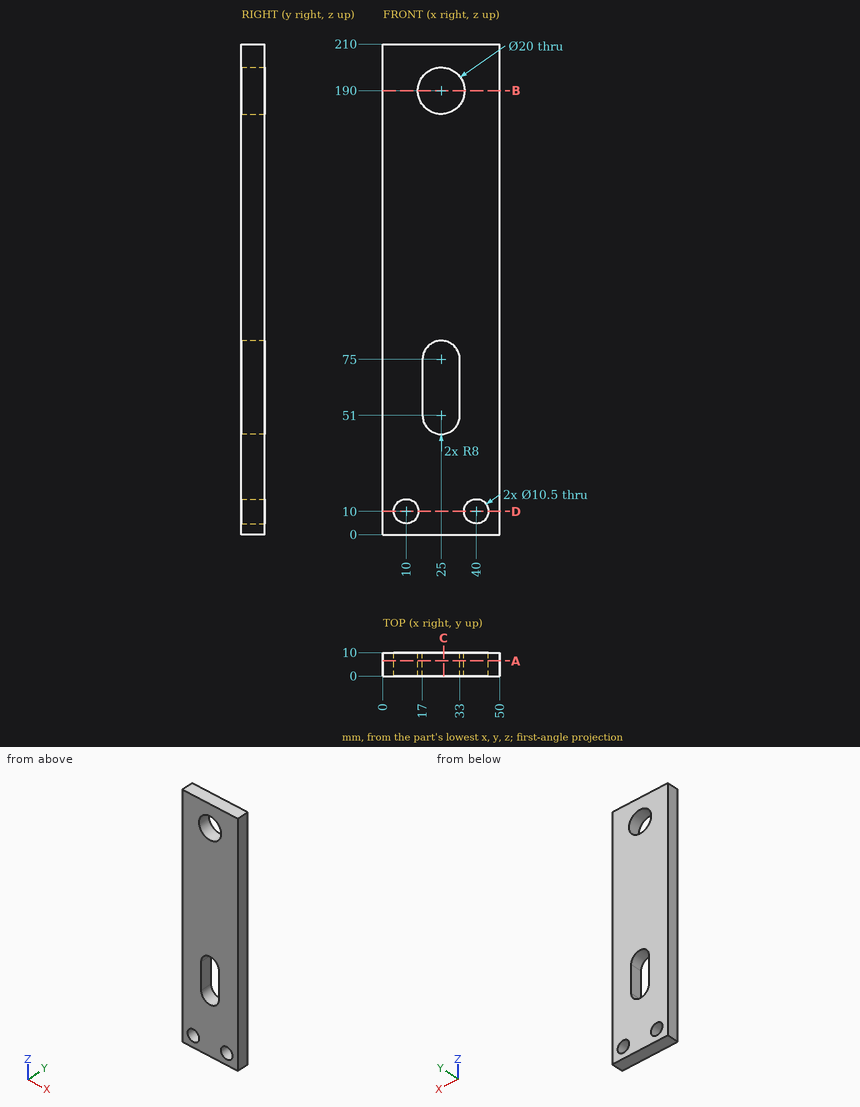
Answer from the drawing. Dimensions are ordinates in mm from the lowest x, y and z of the part. Give positions to 0.01 mm unless a question says otherwise; leave off trailing zeros. Loops run counter-clockwise (first coordinate to the right, second up) from the corner with the lowest first, then second, coordinate; pieces in that order, holes last. Notation, with made-up numbers: (-2, 84.5) -> (6, 84.5) arc R18 ccw to (6, 97.5) -> close; hole circle Ø2 at (35.25, 80.5). An arc over 180 degrees is marked (long way). One line per question, with ' | ' between items. Start each with the question number.
1) Section B-B, the plane z = 190 is taken. Determine the outline of the cut face in (x, y), then the cut area to 3 significant figures.
2) Section D-D, the plane z = 10 is taken. Determine the outline of the cut face in (x, y), then the cut area to 3 significant figures.
3) Straight lines are drawn through the part: L1, parallel to Z at x = 25, y = 7.25; L2, parallel to Z at x = 10, y = 7.75; L3, parallel to Z at x = 24, y = 1.5. For each, find the intervals that lie inside material, in ascending order.
4) Section C-C, the plane x = 26 is taken. Determine the outline of the cut face in (y, z), then the cut area to 3 significant figures.
5) Section A-A, the plane y = 6.5 is taken. Determine the outline of the cut face in (x, z).
Resolved:
1) outline: (0, 0) -> (15, 0) -> (15, 10) -> (0, 10) -> close; (35, 0) -> (50, 0) -> (50, 10) -> (35, 10) -> close | area: 300 mm2
2) outline: (0, 0) -> (4.75, 0) -> (4.75, 10) -> (0, 10) -> close; (15.25, 0) -> (34.75, 0) -> (34.75, 10) -> (15.25, 10) -> close; (45.25, 0) -> (50, 0) -> (50, 10) -> (45.25, 10) -> close | area: 290 mm2
3) L1: 0 to 43, 83 to 180, 200 to 210 | L2: 0 to 4.75, 15.25 to 210 | L3: 0 to 43.06, 82.94 to 180.05, 199.95 to 210
4) outline: (0, 0) -> (10, 0) -> (10, 43.06) -> (0, 43.06) -> close; (0, 82.94) -> (10, 82.94) -> (10, 180.05) -> (0, 180.05) -> close; (0, 199.95) -> (10, 199.95) -> (10, 210) -> (0, 210) -> close | area: 1,500 mm2
5) outline: (0, 0) -> (50, 0) -> (50, 210) -> (0, 210) -> close; hole circle Ø10.5 at (10, 10); hole circle Ø20 at (25, 190); hole (17, 51) arc R8 ccw to (33, 51) -> (33, 75) arc R8 ccw to (17, 75) -> close; hole circle Ø10.5 at (40, 10)
